Autodesk Inventor part; units mm, degrees
ref_plane "YZ Plane" through (0, 0, 0) normal (1, 0, 0) x (0, 1, 0)
ref_plane "XZ Plane" through (0, 0, 0) normal (0, 1, 0) x (-1, 0, 0)
ref_plane "XY Plane" through (0, 0, 0) normal (0, 0, 1) x (1, 0, 0)
sketch "Sketch1" plane through (0, 0, 0) normal (0, 1, 0) x (-1, 0, 0)
  line L0 (0, 0) -> (-37.5, 0)
  line L1 (-37.5, 0) -> (-37.5, 37.5)
  line L2 (-37.5, 37.5) -> (0, 37.5)
  line L3 (0, 37.5) -> (0, 0)
  circle A0 centre (-18.75, 18.75) radius 15.75
  point P0 (-18.75, 0)
  dimension "d0" = 37.5
  dimension "d1" = 37.5
  dimension "d2" = 18.75
  dimension "d3" = 18.75
  dimension "d4" = 31.5
extrude "Extrusion1" add sketch "Sketch1" against normal blind 20
sketch "Sketch3" plane through (0, 0, 37.5) normal (0, 0, 1) x (1, 0, 0)
  circle A0 centre (20.5, -10) radius 4.5
  point P0 (0, 0)
  dimension "d8" = 9
extrude "Extrusion2" cut sketch "Sketch3" against normal blind 5
sketch "Sketch4" plane through (37.5, 0, 0) normal (0, 0, -1) x (-1, 0, 0)
  circle A0 centre (17, -10) radius 4.5
  circle A1 centre (17, -10) radius 2.5
  point P0 (37.5, 0)
  dimension "d11" = 5
extrude "Extrusion3" cut sketch "Sketch4" against normal blind 5 contours A1
sketch "Sketch5" plane through (0, 0, 37.5) normal (0, 0, 1) x (1, 0, 0)
  line L0 (37.5, 0) -> (0, 0)
  line L1 (0, -20) -> (37.5, -20)
  line L2 (0, 0) -> (37.5, 0)
  line L3 (37.5, 0) -> (37.5, -20)
  line L4 (37.5, -20) -> (0, -20)
  line L5 (0, -20) -> (0, 0)
  line L6 (0, 0) -> (0, -20)
  line L7 (0, 0) -> (37.5, 0)
  line L8 (37.5, 0) -> (37.5, -20)
  line L9 (37.5, -20) -> (0, -20)
  line L10 (0, -20) -> (0, 0)
  circle A0 centre (20.5, -10) radius 4.5
extrude "Extrusion4" add sketch "Sketch5" along normal blind 2
sketch "Sketch6" plane through (0, 0, 39.5) normal (0, 0, 1) x (1, 0, 0)
  line L0 (0, 0) -> (0, -20)
  line L1 (0, -20) -> (37.5, -20)
  line L2 (0, 0) -> (37.5, 0)
  line L3 (37.5, 0) -> (37.5, -20)
  line L4 (37.5, -20) -> (0, -20)
  line L5 (0, -20) -> (0, 0)
  circle A0 centre (20.5, -10) radius 2.5
extrude "Extrusion5" add sketch "Sketch6" along normal blind 5
equation "\"d0\" = d1"
properties part number "welco mount v03"
Work out the finished part from the listing and answer in its coordinate system (mm). A direction names the side the tool comes from. Give positions to 0.01 mm unless a question says otherwise; leave off trailing zeros. Write each loop counter-clockwise with the first axis right and the second up, starting at its lowest first coordinate (ties: lowest second). Pieces come first, ordered by that corner, then holes.
(1) Which of the six approach directions +Z, -Z, +X, -X, +Y, -Y give full straight-line access (tool end or side, diameter ignored) to faces 4 (the flat face through (22.4, -11.9, 39.5)), 5 (the flat face through (18, -12, 44.5))?
Final values:
face 4: none
face 5: +Z, +X, -X, +Y, -Y
(2) Straight lines are drawn through the part: line 1 (Y direction, x = 20.5, z = 41.95); line 2 (X direction, y = -10, z = 35); line 3 (Y direction, x = 20.5, z = 37.5). For each, find the intervals that lie inside material, in ascending order.
Final values:
line 1: y = -20 to -12.5, -7.5 to 0
line 2: x = 0 to 16, 25 to 37.5
line 3: y = -20 to -14.5, -5.5 to 0
(3) The part is cut by section A-A on z = 18.75. Write down the section's boundary in (x, y), plus the area to 3 significant figures.
Final values:
outline: (0, -20) - (3, -20) - (3, 0) - (0, 0) - close; (34.5, -20) - (37.5, -20) - (37.5, 0) - (34.5, 0) - close
area: 120 mm2
(4) The mould has two halves that part along Y. Classify faces 1 (the flat face through (18, -12, 0)), 2 (the flat face through (18, 0, 37)), 3 (the cylindrical face through (23, -10, 2)): pulls with the +Y half, pulls with the -Y half, needs draft (parallel to the pull), parting line crosses it, or undercut.
Final values:
face 1: needs draft
face 2: pulls with the +Y half
face 3: undercut
(5) The part is cut by section D-D on z = 41. Write down the section's boundary in (x, y), plus the area to 3 significant figures.
Final values:
outline: (0, -20) - (37.5, -20) - (37.5, 0) - (0, 0) - close; hole circle Ø5 at (20.5, -10)
area: 730 mm2
(6) The part is cut by section B-B on y = -16.25. Write down the section's boundary in (x, z).
Final values:
outline: (0, 0) - (37.5, 0) - (37.5, 44.5) - (0, 44.5) - close; hole circle Ø31.5 at (18.75, 18.75)
(7) The part is cut by section C-C on x = 24. Write down the section's boundary in (y, z), plus the area to 3 significant figures.
Final values:
outline: (-20, 0) - (0, 0) - (0, 3.9) - (-20, 3.9) - close; (-20, 33.6) - (-12.83, 33.6) - (-12.83, 39.5) - (-7.17, 39.5) - (-7.17, 33.6) - (0, 33.6) - (0, 44.5) - (-20, 44.5) - close
area: 263 mm2
